Geometry: final body of the model. Coordinates: model frame, mm. Face numbers are marked on the shaded views. A direction names the side the tool comes from. Coordinates: 2 decimals unless noted, no trailing zeros. Loops run counter-clockwise (first coordinate to the right, second up) from the corner with the lowest first, then second, coordinate; pieces in that order, holes last. Notation, with made-up numbers: (52.5, -14) - (78.5, -14) arc R33 ccw to (78.5, 16) - close; hole circle Ø11 at (80.5, 40). An arc over 180 degrees is marked (long way). Answer in a Markdown table with one row per item.
Solid Edge part; units mm, degrees
sketch "Sketch1" plane through (0, 0, 0) normal (0, 0, 1) x (1, 0, 0)
  circle A0 centre (0, 0) radius 37.5
extrude "Extrusionsausprägung_1" add sketch "Sketch1" along normal blind 6
hole "Bohrung_1" at (-19.44, 19.4509, 6) direction (0, 0, -1) diameter 10 depth 5
hole "Hole1" at (19.4509, 19.44, 6) direction (0, 0, -1) diameter 10 depth 5
hole "Hole2" at (19.44, -19.4509, 6) direction (0, 0, -1) diameter 10 depth 5
hole "Hole3" at (-19.4509, -19.44, 6) direction (0, 0, -1) diameter 10 depth 5
sketch "Sketch2" plane through (0, 0, 0) normal (0, -1, 0) x (1, 0, 0)
  line L0 (-2.5, 0) -> (2.5, 0)
  line L1 (2.5, 0) -> (2, -1.5)
  line L2 (2, -1.5) -> (-2, -1.5)
  line L3 (-2, -1.5) -> (-2.5, 0)
  dimension "D1" = 2
  dimension "D2" = 2.5
extrude "Extrusionsausprägung_2" add sketch "Sketch2" along normal mid plane 50
hole "Bohrung_5" at (0, 30, 6) direction (0, 0, -1) diameter 3.6 end up to next counterbore diameter 6.5 counterbore depth 3.5
hole "Hole4" at (0, -30, 6) direction (0, 0, -1) diameter 3.6 end up to next counterbore diameter 6.5 counterbore depth 3.5
sketch "Sketch3" plane through (0, 0, 6) normal (0, 0, 1) x (-1, 0, 0)
  line L0 (34, -6) -> (34, 6)
  arc A0 (34, 6) -> (30, 10) centre (30, 6) ccw
  arc A1 (30, -10) -> (34, -6) centre (30, -6) ccw
  dimension "D1" = 30
revolve "Rotationsausprägung_1" add sketch "Sketch3" angle 360 about axis through (-30, -10, 6) along (0, 1, 0)
mirror "Mirror1" about plane through (0, 0, 0) normal (1, 0, 0) of "Rotationsausprägung_1"
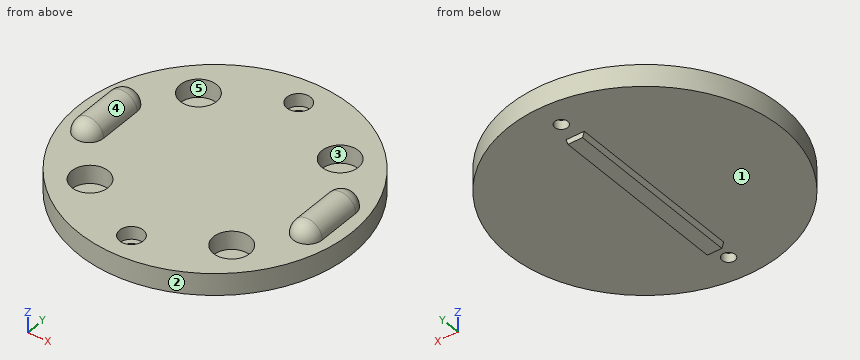
(1) Ray query, probe 1 along Y at (x, z) = (0, 4.45); probe 2 along Y at (x, z) = (0, 1.6); probe 3 along X at (y, z) = (19.44, 2.1). Return the intervals inside material, ascending.
Verdict:
| item | result |
|---|---|
| probe 1 | y = -37.5 to -33.25, -26.75 to 26.75, 33.25 to 37.5 |
| probe 2 | y = -37.5 to -31.8, -28.2 to 28.2, 31.8 to 37.5 |
| probe 3 | x = -32.07 to -24.44, -14.44 to 14.45, 24.45 to 32.07 |
(2) First-contact query: pin 1 Ø2 at (x, z) = (-13.5, 8.5) entering from -Y; pin 2 Ø11 at (x, y) = (-21.5, 19) entering from +Z; pin 3 Ø0.5 at (x, z) = (-0.5, -1) entering from -Y; pin 4 Ø9 at (x, y) = (-19.44, 19.45) entering from -Z. Flat tips, straight axial feed; report the tip coordinate or a pass-through.
Verdict:
| item | result |
|---|---|
| pin 1 | passes through |
| pin 2 | stops at z = 6 |
| pin 3 | stops at y = -25 |
| pin 4 | stops at z = 0 |
(3) Access query for the marked faces 4 and 5. Directions: +Z, -Z, +X, -X, +Y, -Y. A direction counts if a zero-diameter tool reaches every point of the face in a straight line with its end or side. Return the directions, or none.
Verdict:
| item | result |
|---|---|
| face 4 | +Z, +Y, -Y |
| face 5 | +Z |
(4) Cut plane A-A on y = 30. Output: boundary loops of the cut face in (x, z).
Verdict:
| item | result |
|---|---|
| outline | (-22.5, 0) - (-1.8, 0) - (-1.8, 2.5) - (-3.25, 2.5) - (-3.25, 6) - (-22.5, 6) - close; (1.8, 0) - (22.5, 0) - (22.5, 6) - (3.25, 6) - (3.25, 2.5) - (1.8, 2.5) - close |
(5) Cut plane B-B on x = 0. Output: boundary loops of the cut face in (y, z), then the cut area to 4 significant figures.
Verdict:
| item | result |
|---|---|
| outline | (-37.5, 0) - (-31.8, 0) - (-31.8, 2.5) - (-33.25, 2.5) - (-33.25, 6) - (-37.5, 6) - close; (-28.2, 0) - (-25, 0) - (-25, -1.5) - (25, -1.5) - (25, 0) - (28.2, 0) - (28.2, 2.5) - (26.75, 2.5) - (26.75, 6) - (-26.75, 6) - (-26.75, 2.5) - (-28.2, 2.5) - close; (31.8, 0) - (37.5, 0) - (37.5, 6) - (33.25, 6) - (33.25, 2.5) - (31.8, 2.5) - close |
| area | 461.5 mm² |
(6) Cut plane D-D on x = -22.5. Output: boundary loops of the cut face in (y, z).
Verdict:
| item | result |
|---|---|
| outline | (-30, 0) - (30, 0) - (30, 6) - (23.41, 6) - (23.41, 1) - (15.5, 1) - (15.5, 6) - (-15.48, 6) - (-15.48, 1) - (-23.4, 1) - (-23.4, 6) - (-30, 6) - close |
(7) Pull-direction query (Y, two-part tool) for the marked faces 1, 2 and 3; classes: pulls with the +Y half, pulls with the -Y half, needs draft (parallel to the pull), parting line crosses it, or undercut.
Verdict:
| item | result |
|---|---|
| face 1 | needs draft |
| face 2 | parting line crosses it |
| face 3 | undercut |
(8) Cut plane C-C on z = 3.5. Output: boundary loops of the cut face in (x, y).
Verdict:
| item | result |
|---|---|
| outline | circle Ø75 at (0, 0); hole circle Ø10 at (-19.45, -19.44); hole circle Ø10 at (-19.44, 19.45); hole circle Ø6.5 at (0, -30); hole circle Ø6.5 at (0, 30); hole circle Ø10 at (19.44, -19.45); hole circle Ø10 at (19.45, 19.44) |
